from build123d import *

# Parameters (mm, degrees)
SKETCH1_R           = 110
SKETCH1_R_2         = 1.768866344
SKETCH1_R_3         = 1.493909961
SKETCH1_R_4         = 1.739193209
SKETCH1_W           = 20
SKETCH1_H           = 5
SKETCH1_W_2         = 5
SKETCH1_H_2         = 30
BOSS_EXTRUDE1_DEPTH = 5


with BuildPart() as part:
    # Sketch1 → Boss-Extrude1 (new body)
    with BuildSketch(Plane.XY):
        Circle(SKETCH1_R)
        with Locations((-11.691342951, 6.75)):
            Circle(SKETCH1_R_2, mode=Mode.SUBTRACT)
        with Locations((11.691342951, 6.75)):
            Circle(SKETCH1_R_3, mode=Mode.SUBTRACT)
        with Locations((0, -13.5)):
            Circle(SKETCH1_R_4, mode=Mode.SUBTRACT)
        with Locations((-20, 57.5)):
            Rectangle(SKETCH1_W, SKETCH1_H, mode=Mode.SUBTRACT)
        with Locations((20, 57.5)):
            Rectangle(SKETCH1_W, SKETCH1_H, mode=Mode.SUBTRACT)
        with Locations((37.5, 35)):
            Rectangle(SKETCH1_W_2, SKETCH1_H_2, mode=Mode.SUBTRACT)
        with Locations((37.5, -35)):
            Rectangle(SKETCH1_W_2, SKETCH1_H_2, mode=Mode.SUBTRACT)
        with Locations((20, -57.5)):
            Rectangle(SKETCH1_W, SKETCH1_H, mode=Mode.SUBTRACT)
        with Locations((-20, -57.5)):
            Rectangle(SKETCH1_W, SKETCH1_H, mode=Mode.SUBTRACT)
        with Locations((-37.5, -35)):
            Rectangle(SKETCH1_W_2, SKETCH1_H_2, mode=Mode.SUBTRACT)
        with Locations((-37.5, 35)):
            Rectangle(SKETCH1_W_2, SKETCH1_H_2, mode=Mode.SUBTRACT)
    extrude(amount=BOSS_EXTRUDE1_DEPTH)


solid = part.part
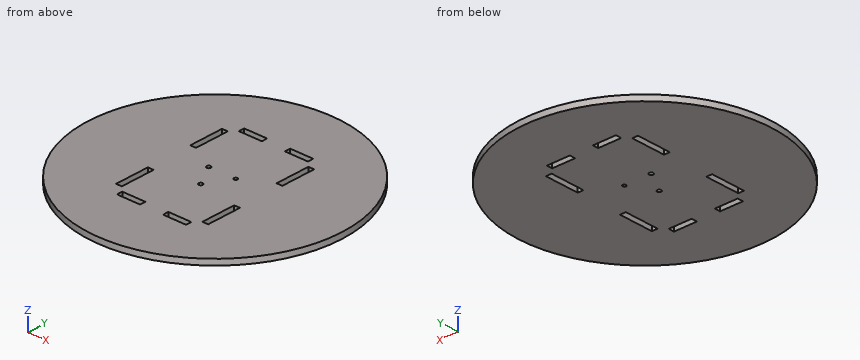
Geometry check sheet. Reference: the model listing, model coordinates, mm. Round coordinates to 2 decimals unless told otherwise and drop trailing zeros. Write each loop counter-clockwise with the first axis right and the second up, starting at its lowest first coordinate (ties: lowest second). Pieces come first, ordered by that corner, then holes.
Item 1: Material ranges on line 1 along Y through (x, z) = (0, 1.8); line 2 along Y through (x, z) = (19, 1.85); line 3 along X through (y, z) = (57.5, 2.25) (3 decimals), recorded low to high.
Determined:
line 1: y = -110 to -15.24, -11.76 to 110
line 2: y = -108.35 to -60, -55 to 55, 60 to 108.35
line 3: x = -93.775 to -30, -10 to 10, 30 to 93.775
Item 2: Section check D-D (x = 77.5). Record the boundary of the cut face in (y, z), plus the area to 3 significant figures.
Determined:
outline: (-78.06, 0) - (78.06, 0) - (78.06, 5) - (-78.06, 5) - close
area: 781 mm2
Item 3: Go/stop test with flat-tipped pins: pin 1 Ø1.5 at (y, z) = (-41.5, 1.5) entering from -X; pin 2 Ø2.5 at (y, z) = (-57, 3) entering from +X; pin 3 Ø2.5 at (x, z) = (-21.5, 2.5) entering from +Y. Record where each tip stops, or that it passes through.
Determined:
pin 1: stops at x = -102.17
pin 2: stops at x = 94.83
pin 3: stops at y = 108.12
Item 4: Section check A-A (y = 24.5). Record the boundary of the cut face in (x, z).
Determined:
outline: (-107.24, 0) - (-40, 0) - (-40, 5) - (-107.24, 5) - close; (-35, 0) - (35, 0) - (35, 5) - (-35, 5) - close; (40, 0) - (107.24, 0) - (107.24, 5) - (40, 5) - close
Item 5: Section check C-C (y = -25). Record the boundary of the cut face in (x, z).
Determined:
outline: (-107.12, 0) - (-40, 0) - (-40, 5) - (-107.12, 5) - close; (-35, 0) - (35, 0) - (35, 5) - (-35, 5) - close; (40, 0) - (107.12, 0) - (107.12, 5) - (40, 5) - close
Item 6: Section check B-B (z = 2.45). Give the number of separate pieces and of enclosed holes in the cut face, plus the area to 3 significant figures.
Determined:
separate pieces: 1
enclosed holes: 11
area: 37,000 mm2
